For this review, take the finished solid that the model builds, in its own axes (mm). A direction names the side the tool comes from. Round coordinates to 2 decimals unless told otherwise and drop trailing zeros. Loops run counter-clockwise (first coordinate to the right, second up) from the corner with the lowest first, then second, coordinate; pieces in that order, holes last.
1) Insertion check: pin 1 (1.5 mm diameter, centred on x = -3.5, z = 7.5, fed in from +Y); pin 2 (2 mm diameter, centred on y = 20.5, z = 8, fed in from -X); pin 3 (5.5 mm diameter, centred on y = 23.5, z = 10, fed in from +X); pin 4 (4 mm diameter, centred on x = -9.59, z = 4.6, fed in from +Y). Each pin has a flat end and moves straight along its axis. Give the tip position at first contact, or say it passes through.
2) Take a section at B-B (y = 21). State the section outline as (x, z) points.
3) Tool access review of faces 4 (the flat face through (23.9, 27.252, 10.1)), 5 (the flat face through (36.347, 3, 10)), 6 (the flat face through (-7, 18.402, 10)): name each direction out of +Z, -Z, +X, -X, +Y, -Y from which nothing blocks a thin tool from reaching the whole face with its end or side.
4) Mouldability with a two-part tool opening along Z and no side actions: class faces 1 (the cylindrical face through (-7.37, 17.17, 15.07)), 2 (the flat face through (16, 8, 20)), 3 (the flat face through (-11.153, 17, 18)) as pulls with the +Z half, pulls with the -Z half, needs draft (parallel to the pull), parting line crosses it, or undercut.
5) Take a section at C-C (x = -0.5). State the section outline as (y, z) points.
6) Wall thickness on L1, parallel to X at y = 25, z = 1.25; L2, parallel to X at y = 17.3, z = 4.6; L3, parallel to Y at x = -6, z = 8.5: over which ranges is each line inside the solid? List them lowest first.
```python
from build123d import *

# Parameters (mm, degrees)
EXTRUDE_1_DEPTH     = 20
SKETCH_2_R          = 2.225
CUT_EXTRUDE_4_DEPTH = 5
SKETCH_3_R          = 2.225
CUT_EXTRUDE_5_DEPTH = 5
SKETCH_4_R          = 5
EXTRUDE_3_DEPTH     = 1.7
CHAMFER_3_SIZE      = 1.7
SKETCH_5_R          = 3
EXTRUDE_4_DEPTH     = 4.25


with BuildPart() as part:
    # 草圖1 → 填料-伸長1 (new body)
    with BuildSketch(Plane.XY):
        Polygon((-4.152823353, 15.901861702), (-4.152823353, -10.448138298), (36.347176647, -10.448138298), (36.347176647, 15.901861702), (43.347176647, 15.901861702), (43.347176647, 18.401861702), (36.347176647, 18.401861702), (36.347176647, 25.551861702), (-4.152823353, 25.551861702), (-4.152823353, 18.401861702), (-11.152823353, 18.401861702), (-11.152823353, 15.901861702), align=None)
    extrude(amount=EXTRUDE_1_DEPTH)

    # 草圖2 → 除料-伸長4 (cut)
    with BuildSketch(Plane(origin=(0, 18.401861702, 0), x_dir=(1, 0, 0), z_dir=(0, 1, 0))):
        with Locations((41.785976647, -4.6)):
            Circle(SKETCH_2_R)
        with Locations((41.785976647, -15)):
            Circle(SKETCH_2_R)
    extrude(amount=-CUT_EXTRUDE_4_DEPTH, mode=Mode.SUBTRACT)

    # 草圖3 → 除料-伸長5 (cut)
    with BuildSketch(Plane(origin=(0, 18.401861702, 0), x_dir=(1, 0, 0), z_dir=(0, 1, 0))):
        with Locations((-9.592823353, -4.6)):
            Circle(SKETCH_3_R)
        with Locations((-9.592823353, -15)):
            Circle(SKETCH_3_R)
    extrude(amount=-CUT_EXTRUDE_5_DEPTH, mode=Mode.SUBTRACT)

    # 草圖4 → 填料-伸長3 (add)
    with BuildSketch(Plane(origin=(0, 25.551861702, 0), x_dir=(1, 0, 0), z_dir=(0, 1, 0))):
        with Locations(Location((27.139664618, -10, 0), (0, 0, 180))):
            Circle(SKETCH_4_R)
    extrude(amount=EXTRUDE_3_DEPTH)

    # 導角3
    chamfer_3_edges = [part.edges().sort_by_distance(p)[0] for p in [
        (32.139664618, 25.551861702, 10),
    ]]
    chamfer(chamfer_3_edges, length=CHAMFER_3_SIZE - 0.0001)  # a hair under: the kernel refuses the full size

    # 草圖5 → 填料-伸長4 (add)
    with BuildSketch(Plane(origin=(0, 27.251861702, 0), x_dir=(1, 0, 0), z_dir=(0, 1, 0))):
        with Locations(Location((27.139664618, -10, 0), (0, 0, 180))):
            Circle(SKETCH_5_R)
    extrude(amount=EXTRUDE_4_DEPTH)


solid = part.part
```
Response:
1. pin 1: stops at y = 25.55
1. pin 2: stops at x = -4.15
1. pin 3: stops at x = 36.35
1. pin 4: passes through
2. outline: (-4.15, 0) - (36.35, 0) - (36.35, 20) - (-4.15, 20) - close
3. face 4: +Y
3. face 5: +Z, -Z, +X, -Y
3. face 6: +Z, -Z, -X, +Y
4. face 1: undercut
4. face 2: pulls with the +Z half
4. face 3: needs draft
5. outline: (-10.45, 0) - (25.55, 0) - (25.55, 20) - (-10.45, 20) - close
6. L1: x = -4.15 to 36.35
6. L2: x = -7.37 to 39.56
6. L3: y = 15.9 to 18.4
